```python
from build123d import *

# Parameters (mm, degrees)
SKETCH1_R           = 6
SKETCH1_R_2         = 4.1
BOSS_EXTRUDE1_DEPTH = 2
SKETCH2_R           = 6
SKETCH2_R_2         = 1.75
BOSS_EXTRUDE2_DEPTH = 2
FILLET1_R           = 1


with BuildPart() as part:
    # Sketch1 → Boss-Extrude1 (new body)
    with BuildSketch(Plane.XY):
        Circle(SKETCH1_R)
        Circle(SKETCH1_R_2, mode=Mode.SUBTRACT)
    extrude(amount=BOSS_EXTRUDE1_DEPTH)

    # Sketch2 → Boss-Extrude2 (add)
    with BuildSketch(Plane.XY.offset(2)):
        Circle(SKETCH2_R)
        Circle(SKETCH2_R_2, mode=Mode.SUBTRACT)
    extrude(amount=BOSS_EXTRUDE2_DEPTH)

    # Fillet1
    fillet1_edges = [part.edges().sort_by_distance(p)[0] for p in [
        (-6, 0, 4),
        (-4.1, 0, 0),
    ]]
    fillet(fillet1_edges, radius=FILLET1_R)


solid = part.part
```
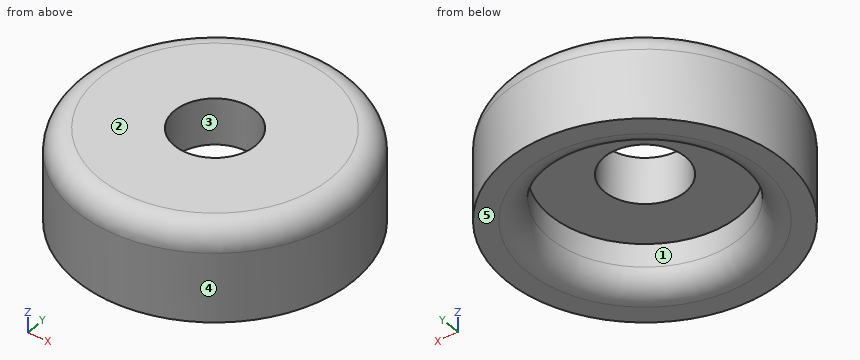
Source: CAD feature listing. Evaluate the final solid. Frame: model axes, mm. Face numbers are marked on the shaded views. A direction names the side the tool comes from. Coordinates: 2 decimals unless noted, no trailing zeros. Loops run counter-clockwise (first coordinate to the right, second up) from the corner with the lowest first, then second, coordinate; pieces in that order, holes last. Notation, with made-up numbers: M -8.5,88 L 40.5,88 A28 ccw 40.5,113 Z; hole C 82,11.5 d8. An arc over 180 degrees is marked long. Put each result on its own line as item: value. Start each with the question number.
1) Cut plane D-D on z = 3.75. Return the cut outline in (x, y).
2) Ray query, L1, parallel to Y at x = 0, z = 2.75; L2, parallel to Y at x = 0, z = 1.8; L3, parallel to Z at x = -2.5, y = -1.5. Return the intervals inside material, ascending. Write a range as from..to.
3) Cut plane A-A on x = 0. Return the cut outline in (y, z), then the cut area to 3 significant figures.
4) Cut plane C-C on z = 2.7. Return the cut outline in (x, y), then the cut area to 3 significant figures.
5) Pull-direction query (Y, two-part tool) for the marked faces 3, 4 and 5; classes: pulls with the +Y half, pulls with the -Y half, needs draft (parallel to the pull), parting line crosses it, or undercut.
6) Reachability of the marked faces 1 and 2 from +Z, -Z, +X, -X, +Y, -Y: full face, straight path, thin tool, end or side. Return the list, or none.
7) Contact query for flat-ended pins moving along their axis: pin 1 Ø4 at (x, y) = (-0.5, -2) entering from -Z; pin 2 Ø1 at (y, z) = (-4.5, 2) entering from +X. Output: stop coordinate, or through.
The answers:
1. outline: C 0,0 d11.32; hole C 0,0 d3.5
2. L1: y = -6..-1.75, 1.75..6
2. L2: y = -6..-4.1, 4.1..6
2. L3: z = 2..4
3. outline: M -6,0 L -5.1,0 A1 ccw -4.1,1 L -4.1,2 L -1.75,2 L -1.75,4 L -5,4 A1 ccw -6,3 Z; M 1.75,2 L 4.1,2 L 4.1,1 A1 ccw 5.1,0 L 6,0 L 6,3 A1 ccw 5,4 L 1.75,4 Z
3. area: 23.7 mm²
4. outline: C 0,0 d12; hole C 0,0 d3.5
4. area: 103 mm²
5. face 3: undercut
5. face 4: parting line crosses it
5. face 5: needs draft
6. face 1: -Z
6. face 2: +Z, +X, -X, +Y, -Y
7. pin 1: stops at z = 2
7. pin 2: stops at x = 4.47
